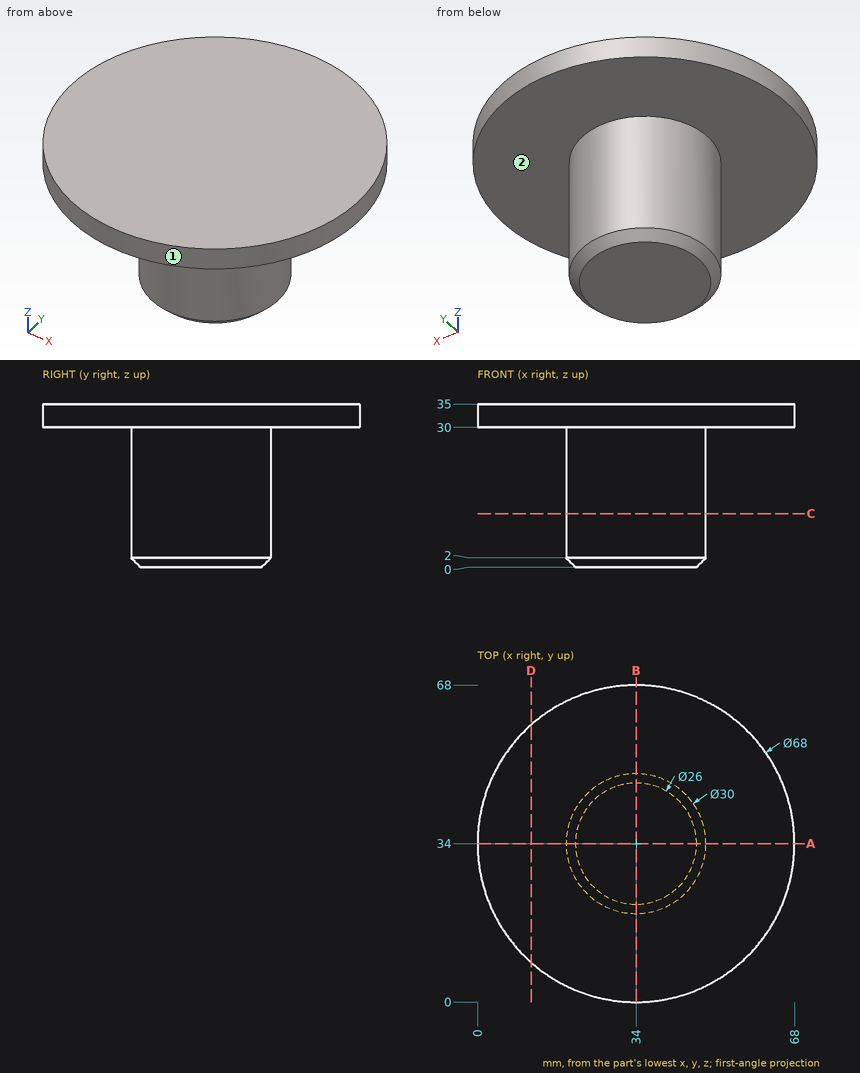
For this review, use the dimensioned drawing (mm, ordinates from the lowest corner) and the shaded views. A direction names the side the tool comes from. Give positions to 0.01 mm unless a question says otherwise; leave off trailing zeros. Order: outer loops, then holes, each group sorted by start corner. A loop starts at its lowest first (then second) coordinate and runs counter-clockwise, first axis right, second up. Notation, with made-up numbers: (-5.5, -25.75) - (35.5, -25.75) arc R7 cw to (35.5, -15.75) - close; hole circle Ø5 at (26, -4). An arc over 180 degrees is marked (long way). Use CSV: the item, a comma, the result in double quotes. Start each with the question number.
Q1. Tool access review of the marked faces 1 and 2: name each direction out of +Z, -Z, +X, -X, +Y, -Y from which nothing blocks a thin tool from reaching the whole face with its end or side.
Q2. To check wall thickness, follow line 1 along Z through (x, y) = (9, 18); line 2 along Y through (x, z) = (23, 25); line 3 along X through (y, z) = (43.5, 32). State the ranges of each line that lie inside material, in increasing order. Write a range as [from, to].
Q3. Clearance check with flat-ended pins moving along their axes: pin 1 Ø5 at (x, z) = (22.5, 6.5) entering from +Y; pin 2 Ø5 at (x, z) = (19, 20.5) entering from -Y; pin 3 Ø6 at (x, z) = (45, 20) entering from -Y. State where each tip first meets the part, or that it passes through.
Q4. We need section D-D, the plane x = 11.5. Write out the cut boundary in (y, z).
Q5. We need section A-A, the plane y = 34. Write out the cut boundary in (x, z), and give its area (3 significant figures).
Q6. We need section C-C, the plane z = 11.5. Write out the cut boundary in (x, y), and give its area (3 significant figures).
Outcome:
1,face 1,"+Z, -Z"
1,face 2,"-Z"
2,line 1,"z = [30, 35]"
2,line 2,"y = [23.8, 44.2]"
2,line 3,"x = [1.35, 66.65]"
3,pin 1,"stops at y = 46"
3,pin 2,"stops at y = 25.71"
3,pin 3,"stops at y = 21.31"
4,outline,"(8.51, 30) - (59.49, 30) - (59.49, 35) - (8.51, 35) - close"
5,outline,"(0, 30) - (19, 30) - (19, 2) - (21, 0) - (47, 0) - (49, 2) - (49, 30) - (68, 30) - (68, 35) - (0, 35) - close"
5,area,"1,240 mm^2"
6,outline,"circle Ø30 at (34, 34)"
6,area,"707 mm^2"
